```python
from build123d import *

# Parameters (mm, degrees)
SKETCH1_W              = 10
SKETCH1_H              = 24.07430416
REVOLVE2_ANGLE         = 180
BOSS_EXTRUDE1_START    = 6
SKETCH1_7_W            = 39.916856905
SKETCH1_7_H            = 14.839467349
BOSS_EXTRUDE1_DEPTH    = 3
CUT_REVOLVE2_START     = -19.078784028
CUT_REVOLVE2_OUTLINE_W = 24.07430416
CUT_REVOLVE2_OUTLINE_H = 7
CUT_REVOLVE2_DEPTH     = 39.078784028


with BuildPart() as part:
    # Sketch1 → Revolve2 (revolve)
    with BuildSketch(Plane.XY):
        with Locations((15, 6.197684731)):
            Rectangle(SKETCH1_W, SKETCH1_H)
    revolve(axis=Axis((0, -3.039467349, 0), (0, -1, 0)), revolution_arc=REVOLVE2_ANGLE)

    # Sketch1<7> → Boss-Extrude1 (add)
    with BuildSketch(Plane.XY.offset(BOSS_EXTRUDE1_START)):
        with Locations((38.608341788, 1.580266325)):
            Rectangle(SKETCH1_7_W, SKETCH1_7_H)
    extrude(amount=BOSS_EXTRUDE1_DEPTH)

    # Cut-Revolve2: read off the stored shape, not the designer's step
    # Cut-Revolve2 outline → Cut-Revolve2 (cut)
    with BuildSketch(Plane(origin=(0, 0, 0), x_dir=(0, 1, 0), z_dir=(0.9539392014169458, 0, 0.29999999999999993)).offset(CUT_REVOLVE2_START)):
        with Locations((6.197684731, -3.5)):
            Rectangle(CUT_REVOLVE2_OUTLINE_W, CUT_REVOLVE2_OUTLINE_H)
    extrude(amount=CUT_REVOLVE2_DEPTH, mode=Mode.SUBTRACT)


solid = part.part
```
Build history of the part. All positions in model axes, mm. A direction names the side the tool comes from. Give positions to 0.01 mm unless a question says otherwise; leave off trailing zeros. Loops run counter-clockwise (first coordinate to the right, second up) from the corner with the lowest first, then second, coordinate; pieces in that order, holes last.
Item 1: Slice it at A-A, the plane z = 4.5. List the corners of the cut face in (x, y), and give its area (3 significant figures).
Answers follow:
outline: (-19.49, -5.84) - (-8.93, -5.84) - (-8.93, 18.23) - (-19.49, 18.23) - close; (8.93, -5.84) - (14.31, -5.84) - (14.31, 18.23) - (8.93, 18.23) - close
area: 384 mm2
Item 2: Slice it at D-D, the plane z = 15.5. List the corners of the cut face in (x, y), and give its area (3 significant figures).
Answers follow:
outline: (-12.64, -5.84) - (12.64, -5.84) - (12.64, 18.23) - (-12.64, 18.23) - close
area: 609 mm2
Item 3: Pull direction X, two halves, no side cores. Call faces 4 (the face through (-1.321, 6.366, 9.912)), 5 (the face through (8, -5.839, 10)), 6 (the face through (58.567, 1, 7)): released by +X, released by -X, zero draft, split by the parting line, or undercut.
Answers follow:
face 4: undercut
face 5: zero draft
face 6: released by +X
Item 4: Which spindle directions (+Z, -Z, +X, -X, +Y, -Y) get a long thin tool onto all of the face, cutting with end or side? Do faces 1 (the face through (0, 18.235, 12)), 2 (the face through (39, 2, 6)), 3 (the face through (38, 2, 9)). Say none if no direction does.
Answers follow:
face 1: +Z, -Z, +X, -X, +Y
face 2: -Z, +X, +Y, -Y
face 3: +Z, +X, +Y, -Y
Item 5: Flat gauge pins, fed straight in: pin 1 (2.5 mm diameter, centred on x = 35.5, z = 8, fed in from +Y); pin 2 (7.5 mm diameter, centred on x = 38, y = 5, fed in from -Z); pin 3 (3 mm diameter, centred on y = 9, z = 17, fed in from -X); pin 4 (3 mm diameter, centred on x = 8.5, z = 4, fed in from +Y). Where does each tip first touch, or does it go through?
Answers follow:
pin 1: stops at y = 9
pin 2: stops at z = 6
pin 3: stops at x = -12.64
pin 4: stops at y = 18.23
Item 6: Slice it at C-C, the plane x = 38. List the corners of the cut face in (y, z).
Answers follow:
outline: (-5.84, 6) - (9, 6) - (9, 9) - (-5.84, 9) - close
Item 7: Slice it at B-B, the plane y = 7.25. List the corners of the cut face in (x, z).
Answers follow:
outline: (-20, 0) - (-10, 0) arc R10 cw to (9.54, 3) - (19.08, 6) - (58.57, 6) - (58.57, 9) - (18.65, 9) - (18.65, 7.22) arc R20 ccw to start
Item 8: Drill centre lines: line 1 (Y direction, x = 44.5, z = 6.5); line 2 (Z direction, x = 31, y = 5.5); line 3 (X direction, y = 10.75, z = 9). Where is each one in solid material? Low to high.
Answers follow:
line 1: y = -5.84 to 9
line 2: z = 6 to 9
line 3: x = -17.86 to -4.36, 4.36 to 17.86
